Can you work these out from the model? Positions are in its coordinate system, mm. A direction names the side the tool comes from. Give positions to 0.01 mm unless a question says otherwise; leave off trailing zeros. Order: outer loops, then holes, each group sorted by start corner. A loop starts at its lowest first (then second) coordinate and runs counter-clockwise, first axis right, second up. Notation, with made-up numbers: (79.25, -37) - (126.25, -37) arc R31 ccw to (126.25, 1) - close; hole circle Ø9 at (12.5, -4.5). An arc over 180 degrees is marked (long way). Answer as CSV lines item,"result".
```python
from build123d import *

# Parameters (mm, degrees)
EXTRUDE1_DEPTH     = 3
FILLET2_R          = 0.5
CAVITY1_DEPTH      = 1
CAVITY1_START      = 0.75
CAVITY1_2_DEPTH    = 0.25
CUT_EXTRUDE1_START = -1
CUT_EXTRUDE1_DEPTH = 1


# Read off the part's stored shape, not the designer's step: Cavity1
with BuildPart() as part:
    # Sketch1 → Extrude1 (new body)
    with BuildSketch(Plane.XY):
        with BuildLine():
            Line((-9.604686356, -12), (9.604686356, -12))
            ThreePointArc((9.604686356, -12), (11.301742631, -11.622154055), (12.67818599, -10.56))
            ThreePointArc((12.67818599, -10.56), (16.5, 0), (12.67818599, 10.56))
            ThreePointArc((12.67818599, 10.56), (11.301742631, 11.622154055), (9.604686356, 12))
            Line((9.604686356, 12), (-9.604686356, 12))
            ThreePointArc((-9.604686356, 12), (-11.301742631, 11.622154055), (-12.67818599, 10.56))
            ThreePointArc((-12.67818599, 10.56), (-16.5, 0), (-12.67818599, -10.56))
            ThreePointArc((-12.67818599, -10.56), (-11.301742631, -11.622154055), (-9.604686356, -12))
        make_face()
    extrude(amount=EXTRUDE1_DEPTH)

    # Fillet2
    fillet2_edges = [part.edges().sort_by_distance(p)[0] for p in [
        (11.301742631, -11.622154055, 3),
        (16.5, 0, 3),
        (11.301742631, 11.622154055, 3),
        (0, 12, 3),
        (-11.301742631, 11.622154055, 3),
        (-16.5, 0, 3),
        (-11.301742631, -11.622154055, 3),
        (0, -12, 3),
    ]]
    fillet(fillet2_edges, radius=FILLET2_R)

    # Cavity1 outline → Cavity1 (cut)
    with BuildSketch(Plane.XY):
        with BuildLine():
            ThreePointArc((-9.366025404, 10.5), (-9.465925826, 10.258819045), (-9.5, 10))
            Line((-9.5, 10), (-8.996077446, 10))
            Line((-8.996077446, 10), (-8.996077446, 8.00000585))
            Line((-8.996077446, 8.00000585), (-7.996077446, 8.00000585))
            Line((-7.996077446, 8.00000585), (-7.996077446, 10))
            Line((-7.996077446, 10), (-0.5, 10))
            Line((-0.5, 10), (-0.5, 7.000002926))
            Line((-0.5, 7.000002926), (0.5, 7.000002926))
            Line((0.5, 7.000002926), (0.5, 10))
            Line((0.5, 10), (7.996077446, 10))
            Line((7.996077446, 10), (7.996077446, 8.00000585))
            Line((7.996077446, 8.00000585), (8.996077446, 8.00000585))
            Line((8.996077446, 8.00000585), (8.996077446, 10))
            Line((8.996077446, 10), (10.062305899, 10))
            ThreePointArc((10.062305899, 10), (10.470554189, 9.912870929), (10.807661891, 9.666666667))
            ThreePointArc((10.807661891, 9.666666667), (14.5, 0), (10.807661891, -9.666666667))
            ThreePointArc((10.807661891, -9.666666667), (10.470554189, -9.912870929), (10.062305899, -10))
            Line((10.062305899, -10), (-9.5, -10))
            ThreePointArc((-9.5, -10), (-9.465925826, -10.258819045), (-9.366025404, -10.5))
            Line((-9.366025404, -10.5), (10.5, -10.5))
            Line((10.5, -10.5), (10.5, -11))
            Line((10.5, -11), (12.250437667, -11))
            ThreePointArc((12.250437667, -11), (12.47276199, -10.788214869), (12.67818599, -10.56))
            ThreePointArc((12.67818599, -10.56), (16.5, 0), (12.67818599, 10.56))
            ThreePointArc((12.67818599, 10.56), (12.47276199, 10.788214869), (12.250437667, 11))
            Line((12.250437667, 11), (10.5, 11))
            Line((10.5, 11), (10.5, 10.5))
            Line((10.5, 10.5), (-9.366025404, 10.5))
        make_face()
    extrude(amount=CAVITY1_DEPTH, mode=Mode.SUBTRACT)

    # Cavity1 2 outline → Cavity1 2 (cut)
    with BuildSketch(Plane.XY.offset(CAVITY1_START)):
        with BuildLine():
            ThreePointArc((-8.5, 11), (-9, 10.866025404), (-9.366025404, 10.5))
            Line((-9.366025404, 10.5), (10.5, 10.5))
            Line((10.5, 10.5), (10.5, 11))
            Line((10.5, 11), (-8.5, 11))
        make_face()
        with BuildLine():
            Line((-8.5, -11), (10.5, -11))
            Line((10.5, -11), (10.5, -10.5))
            Line((10.5, -10.5), (-9.366025404, -10.5))
            ThreePointArc((-9.366025404, -10.5), (-9, -10.866025404), (-8.5, -11))
        make_face()
    extrude(amount=CAVITY1_2_DEPTH, mode=Mode.SUBTRACT)

    # Sketch2 → Cut-Extrude1 (cut)
    with BuildSketch(Plane(origin=(0, 0, 0), x_dir=(-1, 0, 0), z_dir=(0, 0, -1)).offset(CUT_EXTRUDE1_START)):
        with BuildLine():
            Line((9.604686356, 10.5), (-12.727922061, 10.5))
            ThreePointArc((-12.727922061, 10.5), (-16.5, 0), (-12.727922061, -10.5))
            Line((-12.727922061, -10.5), (9.604686356, -10.5))
            ThreePointArc((9.604686356, -10.5), (10.665346528, -10.263846285), (11.525623627, -9.6))
            ThreePointArc((11.525623627, -9.6), (15, 0), (11.525623627, 9.6))
            ThreePointArc((11.525623627, 9.6), (10.665346528, 10.263846285), (9.604686356, 10.5))
        make_face()
    extrude(amount=CUT_EXTRUDE1_DEPTH, mode=Mode.SUBTRACT)


solid = part.part
```
1) I'm going to push a flat-ended pin straight in: P1, Ø5, axis at x = -9.5, y = 2.5, coming from the -Z side. Where does the tip first touch, or does it pass through?
Answer block:
P1,"z = 1"
2) If we mould it in two halves opening along Z, with no side actions, what happens to faces 1 (the flat face through (0, 0, 3)), 2 (the cylindrical face through (-11.324, -11.612, 1.232)), 3 (the flat face through (-5, 11, 0))? For each: +Z half, -Z half, draft (parallel to the pull), parting line (faces both ways), or undercut.
Answer block:
face 1,"+Z half"
face 2,"draft"
face 3,"-Z half"
3) I want a section at B-B on z = 1.85. Write out the boundary of the cut face in (x, y), plus the area to 3 significant figures.
Answer block:
outline,"(-12.68, -10.56) arc R4 ccw to (-9.6, -12) - (9.6, -12) arc R4 ccw to (12.68, -10.56) arc R16.5 ccw to (12.68, 10.56) arc R4 ccw to (9.6, 12) - (-9.6, 12) arc R4 ccw to (-12.68, 10.56) arc R16.5 ccw to start"
area,"714 mm2"
4) I want a section at A-A on x = 1.5. Write out the boundary of the cut face in (y, z).
Answer block:
outline,"(-12, 0) - (-10.5, 0) - (-10.5, 0.75) - (-11, 0.75) - (-11, 1) - (11, 1) - (11, 0.75) - (10.5, 0.75) - (10.5, 0) - (12, 0) - (12, 2.5) arc R0.5 ccw to (11.5, 3) - (-11.5, 3) arc R0.5 ccw to (-12, 2.5) - close"
5) Which directions (+Z, -Z, +X, -X, +Y, -Y) give clear straight access to the entire face, cutting with the end or side of a thin tool? Please do faces 4 (the flat face through (0, 12, 1)), 5 (the flat face through (0.6, 10.5, 0.4)).
Answer block:
face 4,"+Z, -Z, +X, -X, +Y"
face 5,"-Z, +X"
6) I need wall thicknesses on line 1 along Y through (x, z) = (4.5, 0.8); line 2 along Z through (x, y) = (-14, -1.25); line 3 along Y through (x, z) = (9, 0.35). Which ranges of each line are inside material? Lowest first, please. Write a range as [from, to].
Answer block:
line 1,"[-12, -11], [11, 12]"
line 2,"[1, 3]"
line 3,"[-12, -10.5], [10.5, 12]"
